Autodesk Inventor part; units mm, degrees
ref_plane "YZ Plane" through (0, 0, 0) normal (1, 0, 0) x (0, 1, 0)
ref_plane "XZ Plane" through (0, 0, 0) normal (0, 1, 0) x (-1, 0, 0)
ref_plane "XY Plane" through (0, 0, 0) normal (0, 0, 1) x (1, 0, 0)
sketch "Szkic1" plane through (0, 0, 0) normal (0, 1, 0) x (-1, 0, 0)
  line L0 (0, 8) -> (-30, 8)
  line L1 (-30, 8) -> (-30, -8)
  line L2 (-30, -8) -> (0, -8)
  line L3 (0, -8) -> (0, 8)
  point P0 (0, 0)
  dimension "d0" = 30
  dimension "d1" = 16
  dimension "d18" = 8
extrude "Płyta1" add sketch "Szkic1" along normal blind 2
sketch "Szkic2" plane through (0, 2, 0) normal (0, 1, 0) x (1, 0, 0)
  line L0 (30, -8) -> (30, 8)
  line L1 (30, 5) -> (29.7, 5)
  line L2 (29.7, 5) -> (29.7, -5)
  line L3 (29.7, -5) -> (30, -5)
  line L4 (30, -5) -> (30, 5)
  line L5 (0, 8) -> (30, 8)
  point P0 (0, 0)
  dimension "d3" = 10
  dimension "d4" = 3
  dimension "d5" = 0.3
extrude "Wyciągnięcie proste1" cut sketch "Szkic2" against normal up to next
sketch "Szkic3" plane through (27.7, 2, -5) normal (1, 0, 0) x (0, -1, 0)
  line L0 (0, 9.5) -> (0, 0.5)
  line L1 (0, 0.5) -> (10, 0.5)
  line L2 (10, 0.5) -> (10, 9.5)
  line L3 (10, 9.5) -> (0, 9.5)
edge flange "Kołnierz1" height 10 angle 90 thickness 2 bend radius 2 thickness toward (1, 0, 0) relief round relief width 0.5 relief depth 1 edges at (29.7, 2, 0) wall of the first edge with corners at (27.7, 2, 4.5) (27.7, 2, -4.5) (27.7, -8, -4.5) (27.7, -8, 4.5)
bend "Zagięcie1"
corner "Narożnik1"
sketch "Szkic5" plane through (27.7, -8, -4.5) normal (-1, 0, 0) x (0, 0, 1)
  line L0 (9, 0) -> (0, 0)
  arc A0 (32.5897, -3.6981) -> (-23.5897, -3.6981) centre (4.5, -108.5303) ccw
  line L1 (9.5, 10) -> (12.5, 10)
  line L2 (32.5897, -3.6981) -> (34.9889, 5.2557)
  line L3 (-23.5897, -3.6981) -> (-25.9889, 5.2557)
  line L4 (0, 6) -> (9, 6)
  arc A1 (34.9889, 5.2557) -> (13, 8.9626) centre (4.5, -108.5303) ccw
  arc A2 (-4, 8.9626) -> (-25.9889, 5.2557) centre (4.5, -108.5303) ccw
  line L5 (-4, 8.9626) -> (-4, 4.9626)
  line L6 (-4, 4.9626) -> (13, 4.9626)
  line L7 (13, 4.9626) -> (13, 8.9626)
  circle A3 centre (4.5, -108.5303) radius 113
  line L8 (4.5, 0) -> (4.5, -108.5303)
  point P0 (4.5, 8)
  dimension "d38" = 4
  dimension "d39" = 17
  dimension "d42" = 226
  dimension "d69" = 108.5303
sheet face with bend "Powierzchnia2" sketch "Szkic5" thickness 2 toward (1, 0, 0) bend radius 2 picked at (25.4474, 0.8245) contours A0 L3 A3 L2 | A3 L3 A2 L5 L6 L7 A1 L2
bend "Zagięcie2"
fillet "Zaokrąglenie narożnika1" radius 2 8 edges at (28.7, 0.9626, -8.5) (28.7, -11.6981, -28.0897) (28.7, -11.6981, 28.0897) (28.7, -3.0374, -8.5) (28.7, -2.7443, 30.4889) (28.7, 0.9626, 8.5) (28.7, -3.0374, 8.5) (28.7, -2.7443, -30.4889)
fillet "Zaokrąglenie narożnika2" radius 6 2 edges at (0, 1, 8) (0, 1, -8)
sketch "Szkic6" plane through (27.7, -2, -4.5) normal (-1, 0, 0) x (0, 0, 1)
  point P0 (4.5, 2)
sketch "Szkic7" plane through (27.7, -2, -4.5) normal (-1, 0, 0) x (0, 0, 1)
  line L0 (9, 0) -> (0, 0)
  line L1 (4.5, 0) -> (4.5, -9.6943)
  arc A0 (30.6882, -9.207) -> (-21.6882, -9.207) centre (4.5, -114.5303) ccw
  line L2 (4.5, -6) -> (4.5, -114.5303)
  circle A1 centre (4.5, -114.5303) radius 113
  point P0 (4.5, 2)
  point P1 (24.5, -3.3143)
  point P2 (-15.5, -3.3143)
  dimension "d49" = 20
  dimension "d50" = 20
  dimension "d70" = 108.5303
  dimension "d71" = 226
hole "Otwór1" at (27.7, -5.3143, -20) at (27.7, -5.3143, 20) direction (1, 0, 0) diameter 2.459 end through all
sketch "Szkic8" plane through (0, 0, 0) normal (0, -1, 0) x (1, 0, 0)
  line L0 (30, 5) -> (30, 8)
  point P0 (0, 0)
  point P1 (8, 0)
  point P2 (18, 0)
  dimension "d60" = 8
  dimension "d61" = 10
  dimension "d75" = 12
hole "Otwór2" at (8, 0, 0) at (18, 0, 0) direction (0, 1, 0) diameter 2.459 end through all
chamfer "Faza1" distance 0.3 angle 45 4 edges at (29.7, -5.3143, -21.2295) (29.7, -5.3143, 18.7705) (8, 2, 1.2295) (18, 2, 1.2295)
equation "\"d2\" = Grubość"
equation "\"d9\" = GłębokośćGięciaPodcięcia"
equation "\"d10\" = MinimalnaPozostałość"
equation "\"d11\" = PromieńPrzejścia"
equation "\"d14\" = PromieńGięcia"
equation "\"d15\" = RozmiarPodcięciaNarożnika"
equation "\"d16\" = Wielk_odstępu"
equation "\"d17\" = Rozmiar_promienia_Jacobiego"
equation "\"d31\" = PromieńGięcia"
equation "\"d32\" = SzerokośćGięciaPodcięcia"
equation "\"d34\" = MinimalnaPozostałość"
equation "\"d33\" = GłębokośćGięciaPodcięcia"
equation "\"d35\" = PromieńPrzejścia"
equation "\"PromieńGięcia\" = Grubość"
equation "\"SzerokośćGięciaPodcięcia\" = Grubość"
equation "\"GłębokośćGięciaPodcięcia\" = 0.5 * Grubość"
equation "\"RozmiarPodcięciaNarożnika\" = 4 * Grubość"
equation "\"MinimalnaPozostałość\" = 2 * Grubość"
equation "\"PromieńPrzejścia\" = PromieńGięcia"
equation "\"Rozmiar_promienia_Jacobiego\" = PromieńGięcia"
equation "\"Wielk_odstępu\" = Grubość"
properties part number "NowyKatownik" material "Stal nierdzewna"
Geometry: final body of the model. Coordinates: model frame, mm. A direction names the side the tool comes from. Coordinates: 2 decimals unless noted, no trailing zeros. Loops run counter-clockwise (first coordinate to the right, second up) from the corner with the lowest first, then second, coordinate; pieces in that order, holes last. Notation, with made-up numbers: M 5.25,-33.5 L 23.25,-33.5 A29 cw 23.25,-1.5 Z; hole C 42.25,-14.5 d9. An arc over 180 degrees is marked long. One line per item, written item: value. Start each with the question number.
1) Material intervals for L1, parallel to Z at x = 18, y = 0.8; L2, parallel to X at y = 0.5, z = 0; L3, parallel to X at y = 1.35, z = 0, sorted ascending. Write a range as from..to.
2) Draft query along Z for faces 3 (the cylindrical face through (27.13, -0.6, 0.06)), 4 (the cylindrical face through (28.71, -3.18, -29.77)), 5 (the cylindrical face through (28.714, -2.466, 7.899)). Return one class per face: released by +Z, released by -Z, zero draft, split by the parting line, or undercut.
3) Cut plane A-A (z = -20). Return loops of the section in (x, y), then the cut area to 3 significant figures.
4) Cut plane B-B (z = 0.5). Count the separate pieces of the cut face and the enclosed holes in it, then the cut area to 3 significant figures.
5) Reachability of faces 1 (the flat face through (0, 1, 0)), 2 (the flat face through (28, 1, -5)) from +Z, -Z, +X, -X, +Y, -Y: full face, straight path, thin tool, end or side. Return the list, or none.
6) Cut plane C-C (x = 24). Return loops of the section in (y, z).
7) Pin query (flat end, axial travel): P1, Ø6, axis at y = -6, z = -6, coming from the +X side; P2, Ø1, axis at y = -4.5, z = -6, coming from the -X side; P3, Ø3, axis at x = 19.5, y = -1, coming from the +Z side. Return the tip coordinate at first contact, or that it passes through.
Evaluation:
1. L1: -8..-1.23, 1.23..8
1. L2: 0..6.77, 9.23..16.77, 19.23..28.82
1. L3: 0..6.77, 9.23..16.77, 19.23..27.89
2. face 3: zero draft
2. face 4: released by -Z
2. face 5: undercut
3. outline: M 27.7,-9.86 L 29.7,-9.86 L 29.7,-6.84 L 29.4,-6.54 L 27.7,-6.54 Z; M 27.7,-4.08 L 29.4,-4.08 L 29.7,-3.78 L 29.7,-0.44 L 27.7,-0.44 Z
3. area: 13.8 mm^2
4. separate pieces: 3
4. enclosed holes: 0
4. area: 63.6 mm^2
5. face 1: +Z, -Z, -X, +Y, -Y
5. face 2: +X, +Y
6. outline: M 0,-8 L 2,-8 L 2,8 L 0,8 Z
7. P1: x = 29.7
7. P2: x = 27.7
7. P3: z = 8
